For this review, take the finished solid that the model builds, in its own axes (mm). A direction names the side the tool comes from. Give positions to 0.01 mm unless a question says otherwise; leave off trailing zeros. Write each loop counter-clockwise with the first axis right and the second up, starting at its lowest first coordinate (ties: lowest second). Pieces come first, ordered by that corner, then holes. Notation, with made-up numbers: M 75,2.25 L 86,2.25 A16 cw 86,14.25 Z; hole C 9,42 d5. An arc over 180 degrees is marked long. One line per item, written item: value. Start each with the question number.
Item 1: Mouldability with a two-part tool opening along Y and no side actions: class faces 1 (the face through (8, -2, -3)), 2 (the face through (3.944, 2.325, 4.42)) as released by +Y, released by -Y, zero draft, split by the parting line, or undercut.
Item 2: Clearance check with flat-ended pins moving along their axes: pin 1 Ø0.6 at (y, z) = (-2.5, -4.5) entering from -X; pin 2 Ø5 at (x, y) = (3.5, -2) entering from -Z; pin 3 Ø2 at (x, y) = (-2, 0.5) entering from +Z; pin 4 Ø1 at (x, z) = (3.5, 0) entering from -Y. State where each tip first meets the part, or that it passes through.
Item 3: Tool access review of faces 3 (the face through (0, 4.5, -1.4)), 4 (the face through (0, -3, -4)), 5 (the face through (0, -3, 4)), 6 (the face through (-3, 3, 1)): name each direction out of +Z, -Z, +X, -X, +Y, -Y from which nothing blocks a thin tool from reaching the whole face with its end or side.
Item 4: Consider section C-C, the plane z = -4.25. Write out the cut boundary in (x, y).
Item 5: To check wall thickness, follow probe 1 along Y at (x, z) = (0.5, 3.75); probe 2 along Y at (x, z) = (5.25, 2); probe 3 along Y at (x, z) = (5.5, 0). State the ranges of each line that lie inside material, in increasing order.
Item 6: Consider section A-A, the plane z = 0. Write out the cut boundary in (x, y), and give its area (3 significant figures).
Item 7: Consider section B-B, the plane y = 1. Write out the cut boundary in (x, z).
Item 8: Consider section D-D, the plane y = -4. Write out the cut boundary in (x, z), and give its area (3 significant figures).
```python
from build123d import *
from build123d.topology import SkipClean

# Parameters (mm, degrees)
BASPROSKE_W      = 8
BASPROSKE_H      = 6
TOOTHCUT_DEPTH   = 12.66190379
TEETHCUTS_COUNT  = 10
TEETHCUTS_ANGLE  = 324
HUBNEAONESKE_R   = 3.749
HUBNEARONE_DEPTH = 3.0000508
BORSKE_R         = 3
BORE_DEPTH       = 11.0000508


with BuildPart() as part:
    # BasProSke → Base-Revolve (revolve)
    with BuildSketch(Plane(origin=(0, 0, 0), x_dir=(1, 0, 0), z_dir=(0, 1, 0)), mode=Mode.PRIVATE) as base_revolve_sk:
        with Locations((4, 3)):
            Rectangle(BASPROSKE_W, BASPROSKE_H)
    revolve(base_revolve_sk.sketch.rotate(Axis((-10, 0, 0), (1, 0, 0)), 180), axis=Axis((-10, 0, 0), (1, 0, 0)))

    # TooCutSke → ToothCut (cut, through all)
    with BuildSketch(Plane(origin=(0, 0, 0), x_dir=(0, 0, -1), z_dir=(1, 0, 0))):
        with BuildLine():
            ThreePointArc((0.59278292, 3.701838653), (0, 3.749), (-0.59278292, 3.701838653))
            ThreePointArc((-0.59278292, 3.701838653), (-0.846593509, 4.924114224), (-1.775771316, 5.757784417))
            ThreePointArc((-1.775771316, 5.757784417), (0, 6.0254), (1.775771316, 5.757784417))
            ThreePointArc((1.775771316, 5.757784417), (0.846593509, 4.924114224), (0.59278292, 3.701838653))
        make_face()
    toothcut = extrude(amount=TOOTHCUT_DEPTH, mode=Mode.SUBTRACT)

    # TeethCuts: ToothCut ×10 about axis
    teethcuts_axis = Axis((0, 0, 0), (1, 0, 0))
    for i in range(1, TEETHCUTS_COUNT):
        add(toothcut.rotate(teethcuts_axis, i * TEETHCUTS_ANGLE / (TEETHCUTS_COUNT - 1)), mode=Mode.SUBTRACT)

    # HubNeaOneSke → HubNearOne (add)
    with SkipClean():  # the faces are left unmerged after this step: merging them gives an invalid solid
        with BuildSketch(Plane.ZY):
            Circle(HUBNEAONESKE_R)
        extrude(amount=HUBNEARONE_DEPTH)

    # BorSke → Bore (cut, symmetric)
    with SkipClean():  # the faces are left unmerged after this step: merging them gives an invalid solid
        with BuildSketch(Plane(origin=(0, 0, 0), x_dir=(0, 0, -1), z_dir=(1, 0, 0))):
            with Locations(Location((0, 0, 0), (0, 0, 180))):
                Circle(BORSKE_R)
        extrude(amount=BORE_DEPTH, both=True, mode=Mode.SUBTRACT)


solid = part.part
```
Model answer:
1. face 1: zero draft
1. face 2: undercut
2. pin 1: stops at x = 0
2. pin 2: stops at z = -6
2. pin 3: stops at z = 3.75
2. pin 4: stops at y = -3.75
3. face 3: -Z, -X, +Y
3. face 4: -Z, -X, -Y
3. face 5: +Z, -X, -Y
3. face 6: +Z, -Z, -X, +Y, -Y
4. outline: M 0,-3.65 L 8,-3.65 L 8,-2.16 L 0,-2.16 Z; M 0,-0.74 L 8,-0.74 L 8,0.74 L 0,0.74 Z; M 0,2.16 L 8,2.16 L 8,3.65 L 0,3.65 Z
5. probe 1: y = -3.55 to -1.84, -0.6 to 0.6, 1.84 to 3.55
5. probe 2: y = -5.61 to -3.78, -3.17 to -2.24, 2.24 to 3.17, 3.78 to 5.61
5. probe 3: y = -3.75 to -3, 3 to 3.75
6. outline: M -3,-3.75 L 8,-3.75 L 8,-3 L -3,-3 Z; M -3,3 L 8,3 L 8,3.75 L -3,3.75 Z
6. area: 16.5 mm2
7. outline: M -3,-3.61 L 8,-3.61 L 8,-2.83 L -3,-2.83 Z; M -3,2.83 L 8,2.83 L 8,3.61 L -3,3.61 Z
8. outline: M 0,-2.1 L 8,-2.1 L 8,-0.58 L 0,-0.58 Z; M 0,0.58 L 8,0.58 L 8,2.1 L 0,2.1 Z
8. area: 24.2 mm2
